Autodesk Inventor part; units mm, degrees
ref_plane "YZ Plane" through (0, 0, 0) normal (1, 0, 0) x (0, 1, 0)
ref_plane "XZ Plane" through (0, 0, 0) normal (0, 1, 0) x (-1, 0, 0)
ref_plane "XY Plane" through (0, 0, 0) normal (0, 0, 1) x (1, 0, 0)
sketch "Sketch1" plane through (0, 0, 0) normal (0, 0, 1) x (1, 0, 0)
  line L0 (-651.5983, 84.4921) -> (440.9045, 84.4921)
  line L1 (440.9045, 84.4921) -> (440.9045, -15.5079)
  line L2 (440.9045, -15.5079) -> (-651.5983, -15.5079)
  line L3 (-651.5983, -15.5079) -> (-651.5983, 84.4921)
  line L4 (-651.5983, -15.5079) -> (-899.2765, -81.873)
  point P0 (0, 0)
  dimension "d0" = 100
extrude "Extrusion1" add sketch "Sketch1" against normal blind 50
fillet "Fillet1" radius 3 4 edges at (-105.3469, 84.4921, 0) (-105.3469, 84.4921, -50) (-105.3469, -15.5079, 0) (-105.3469, -15.5079, -50)
shell "Shell1" thickness 3 removed faces 2 at (440.9045, 18.8255, -33.3333) at (-651.5983, 18.8255, -33.3333)
sketch "Sketch2" plane through (0, 0, 0) normal (0, 0, 1) x (1, 0, 0)
  circle A0 centre (377.8245, 22.8431) radius 11.25
  point P0 (0, 0)
extrude "Extrusion2" cut sketch "Sketch2" against normal through all
sketch "Sketch3" plane through (-651.5983, 84.4921, -47) normal (0, 1, 0) x (1, 0, 0)
  line L0 (0, 0) -> (1092.5029, 0)
  line L1 (0, -44) -> (0, 0)
  line L2 (1092.5029, -44) -> (0, -44)
  line L3 (1092.5029, -44) -> (1092.5029, 0)
  line L4 (1092.5029, -44) -> (1016.2926, 0)
  line L5 (0, 0) -> (1092.5029, 0)
  line L6 (1092.5029, -44) -> (1101.6667, -44)
  line L7 (1101.6667, -44) -> (1101.6667, 18.4263)
  line L8 (1101.6667, 18.4263) -> (1016.2926, 18.4263)
  line L9 (1016.2926, 18.4263) -> (1016.2926, 0)
  point P0 (651.5983, -47)
  dimension "d8" = 30
extrude "Extrusion3" cut sketch "Sketch3" against normal through all contours L9 L8 L7 L6 L3 L0 | L0 L3 L4
properties part number "Barra nuevo pivote"
The listing builds one solid part. Answer for the finished solid, in the listing's coordinates (mm). A direction names the side the tool comes from. Give positions to 0.01 mm unless a question says otherwise; leave off trailing zeros. Write each loop counter-clockwise with the first axis right and the second up, starting at its lowest first coordinate (ties: lowest second). Pieces come first, ordered by that corner, then holes. Notation, with made-up numbers: (-32.75, -24) -> (-9.75, -24) arc R5 ccw to (-9.75, -20) -> close; hole circle Ø5 at (-3.75, 59). An arc over 180 degrees is marked (long way). Write item = value, one per line. Start each with the question number.
1) Determine the mould class of faces 1 (the face through (-113, 35, 0)), 2 (the face through (-113, 84.492, -25)), 3 (the face through (-113, 35, -3)), 4 (the face through (-98, -15.508, -25)) for opening direction Y: +Y half, -Y half, draft (parallel to the pull), parting line (faces both ways), or undercut.
2) Straight lines are drawn through the part: line 1 along Z through (x, y) = (269.5, 41); line 2 along Y through (x, z) = (201, -41.5); line 3 along Z through (x, y) = (393, 32.5). For each, find the intervals that lie inside material, in ascending order.
3) Which of the six approach directions +Z, -Z, +X, -X, +Y, -Y give full straight-line access (tool end or side, diameter ignored) to faces 5 (the face through (-98, -12.508, -25)), 6 (the face through (403.333, -13.987, -24.692))?
4) The part is cut by section A-A, the plane x = -585.5. Determine the outline of the cut face in (y, z), and give its area (3 significant figures).
5) The part is cut by section C-C, the plane z = -14. Determine the outline of the cut face in (x, y).
6) Each of these flat-tipped pins is pushed along its axis until it touches: pin 1 (2.5 mm diameter, centred on y = 51, z = -48, fed in from +X); pin 2 (5 mm diameter, centred on y = 54.5, z = -43, fed in from +X). Where does it stop, or does it pass through?
7) The part is cut by section B-B, the plane y = 56. Determine the outline of the cut face in (x, z).
Solutions:
q1.face_1 = draft
q1.face_2 = +Y half
q1.face_3 = undercut
q1.face_4 = -Y half
q2.line_1 = -50 to -47, -3 to 0
q2.line_2 = -15.51 to -12.51, 81.49 to 84.49
q2.line_3 = -3 to 0
q3.face_5 = +X, -X
q3.face_6 = -Z, +X, +Y, -Y
q4.outline = (-15.51, -47) arc R3 ccw to (-12.51, -50) -> (81.49, -50) arc R3 ccw to (84.49, -47) -> (84.49, -3) arc R3 ccw to (81.49, 0) -> (-12.51, 0) arc R3 ccw to (-15.51, -3) -> close; hole (-12.51, -47) -> (81.49, -47) -> (81.49, -3) -> (-12.51, -3) -> close
q4.area = 856 mm²
q5.outline = (-651.6, -15.51) -> (421.85, -15.51) -> (421.85, -12.51) -> (-651.6, -12.51) -> close; (-651.6, 81.49) -> (421.85, 81.49) -> (421.85, 84.49) -> (-651.6, 84.49) -> close
q6.pin_1 = 364.69
q6.pin_2 = through
q7.outline = (-651.6, -50) -> (364.69, -50) -> (364.69, -47) -> (-651.6, -47) -> close; (-651.6, -3) -> (440.9, -3) -> (440.9, 0) -> (-651.6, 0) -> close
